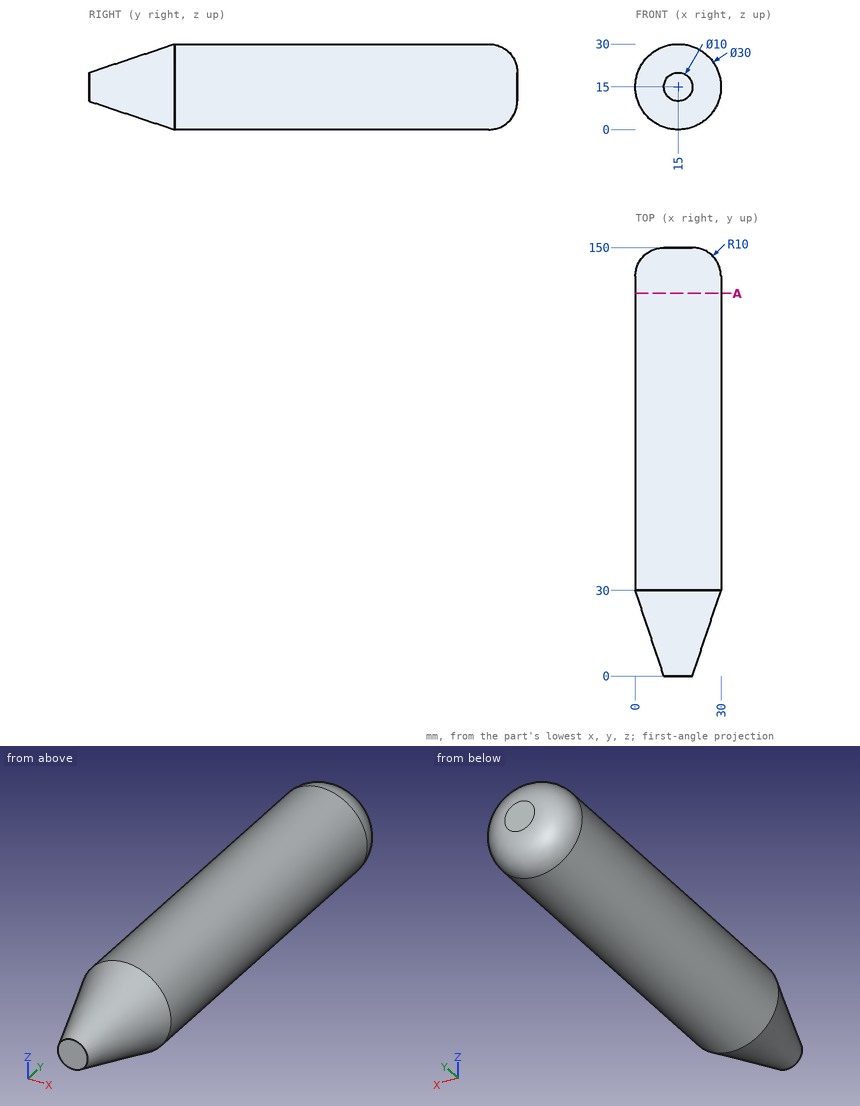
Input: dimensioned drawing with shaded views. Units: mm. Origin: part minimum x, y, z. Round coordinates to 2 decimals unless told otherwise and drop trailing zeros. Loops run counter-clockwise (first coordinate to the right, second up) from the corner with the lowest first, then second, coordinate; pieces in that order, holes last. Notation, with made-up numbers: M 23,-14.5 L 63,-14.5 A15 ccw 63,3.5 Z; hole C 84.5,35 d9. An arc over 180 degrees is marked long. Answer in a Markdown table with one row per item. Add a question column.
1. Section A-A (y = 134). Output: boundary loops of the cut face in (x, z).
2. Contact query for flat-ended pins moving along their axis: pin 1 (4 mm diameter, centred on y = 80.5, z = 25, fed in from +X); pin 2 (2 mm diameter, centred on x = 15.5, y = 19, fed in from +Z); pin 3 (5 mm diameter, centred on y = 115, z = 26.5, fed in from +X). Output: stop coordinate, or through.
3. Ray query, probe 1 along X at (y, z) = (64, 1.5); probe 2 along X at (y, z) = (52.5, 17.5); probe 3 along Z at (x, y) = (20.5, 132). Return the intervals inside material, ascending.
Values follow:
| question | item | result |
|---|---|---|
| 1 | outline | C 15,15 d30 |
| 2 | pin 1 | x = 27.69 |
| 2 | pin 2 | z = 26.66 |
| 2 | pin 3 | x = 27 |
| 3 | probe 1 | 8.46 to 21.54 |
| 3 | probe 2 | 0.21 to 29.79 |
| 3 | probe 3 | 1.04 to 28.96 |
